Geometry: see drawing. Coordinates: mm, zero at the bounding-box minimum. Give positions to 0.01 mm unless a question says otherwise; leave off trailing zeros. Loops run counter-clockwise (first coordinate to the right, second up) from the corner with the lowest first, then second, coordinate; pieces in that order, holes last. Notation, with made-up numbers: M -36,69.5 L 13,69.5 A29 cw 13,91.5 Z; hole C 26,-11 d3. An arc over 180 degrees is marked long. Put each result on its own line as item: value.
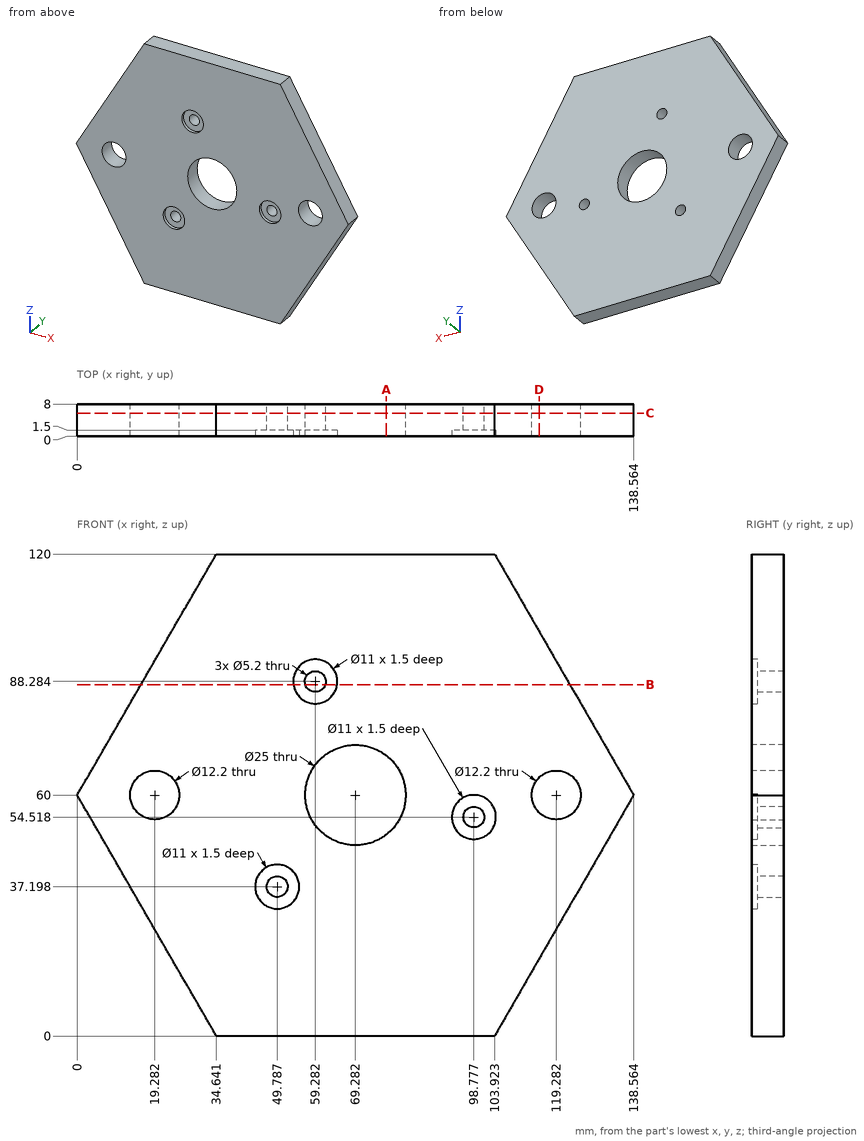
Item 1: Section B-B on z = 87.5. Output: boundary loops of the cut face in (x, y), then the cut area to 3 significant figures.
Output values:
outline: M 15.88,0 L 53.84,0 L 53.84,1.5 L 56.8,1.5 L 56.8,8 L 15.88,8 Z; M 61.76,1.5 L 64.73,1.5 L 64.73,0 L 122.69,0 L 122.69,8 L 61.76,8 Z
area: 806 mm²
Item 2: Section C-C on y = 5.75. Output: boundary loops of the cut face in (x, z) (1 decimal), then the cut area to 3 significant figures.
Output values:
outline: M 0,60 L 34.6,0 L 103.9,0 L 138.6,60 L 103.9,120 L 34.6,120 Z; hole C 19.3,60 d12.2; hole C 49.8,37.2 d5.2; hole C 59.3,88.3 d5.2; hole C 69.3,60 d25; hole C 98.8,54.5 d5.2; hole C 119.3,60 d12.2
area: 11,700 mm²
Item 3: Pin query (flat end, axial travel): pin 1 Ø3 at (x, z) = (59.28, 88.28) entering from +Y; pin 2 Ø2 at (y, z) = (3, 79.5) entering from +X; pin 3 Ø3.5 at (x, z) = (100, 52.5) entering from -Y; pin 4 Ø2 at (y, z) = (6.5, 100.5) entering from +X. Return the tip coordinate at first contact, or that it passes through.
Output values:
pin 1: through
pin 2: x = 127.88
pin 3: y = 1.5
pin 4: x = 115.76
Item 4: Line query: probe 1 along Z at (x, y) = (60, 4) (1 decimal); probe 2 along Z at (x, y) = (115, 6.25) (1 decimal); probe 3 along Z at (x, y) = (122, 3). Output: solid intervals per line, ascending. Write a range as [from, to].
Output values:
probe 1: [0, 51.6], [68.4, 85.8], [90.8, 120]
probe 2: [19.2, 55.7], [64.3, 100.8]
probe 3: [31.31, 54.54], [65.46, 88.69]
Item 5: Section D-D on x = 115. Output: boundary loops of the cut face in (y, z) (1 decimal).
Output values:
outline: M 0,19.2 L 8,19.2 L 8,55.7 L 0,55.7 Z; M 0,64.3 L 8,64.3 L 8,100.8 L 0,100.8 Z
Item 6: Section A-A on x = 77. Output: boundary loops of the cut face in (y, z).
Output values:
outline: M 0,0 L 8,0 L 8,50.17 L 0,50.17 Z; M 0,69.83 L 8,69.83 L 8,120 L 0,120 Z
